```python
from build123d import *

# Parameters (mm, degrees)
BOSS_EXTRUDE1_DEPTH = 3
SKETCH3_W           = 12.065
SKETCH3_H           = 24.13
CUT_EXTRUDE1_DEPTH  = 114.708347838
CUT_EXTRUDE3_DEPTH  = 114.708347838
SKETCH5_R           = 0.8509
CUT_EXTRUDE4_DEPTH  = 114.708347838


with BuildPart() as part:
    # Sketch1 → Boss-Extrude1 (new body)
    with BuildSketch(Plane(origin=(0, 0, 0), x_dir=(1, 0, 0), z_dir=(0, 1, 0))):
        Polygon((0, 0), (0, 20.193), (-3, 20.193), (-3, 32.639), (0, 32.639), (0, 52.832), (41.783, 52.832), (41.783, 55.832), (54.229, 55.832), (54.229, 52.832), (96.012, 52.832), (96.012, 32.639), (99.012, 32.639), (99.012, 20.193), (96.012, 20.193), (96.012, 0), (54.229, 0), (54.229, -3), (41.783, -3), (41.783, 0), align=None)
    extrude(amount=BOSS_EXTRUDE1_DEPTH)

    # Sketch3 → Cut-Extrude1 (cut, through all)
    with BuildSketch(Plane(origin=(0, 3, 0), x_dir=(1, 0, 0), z_dir=(0, 1, 0))):
        with Locations((83.6295, 26.162)):
            Rectangle(SKETCH3_W, SKETCH3_H)
    extrude(amount=-CUT_EXTRUDE1_DEPTH, mode=Mode.SUBTRACT)

    # Sketch4 → Cut-Extrude3 (cut, through all)
    with BuildSketch(Plane(origin=(0, 3, 0), x_dir=(1, 0, 0), z_dir=(0, 1, 0))):
        with BuildLine():
            Line((96.012, 11.43), (96.012, 0))
            Line((96.012, 0), (84.582, 0))
            ThreePointArc((84.582, 0), (87.929769491, 8.082230509), (96.012, 11.43))
        make_face()
    extrude(amount=-CUT_EXTRUDE3_DEPTH, mode=Mode.SUBTRACT)

    # Sketch5 → Cut-Extrude4 (cut, through all)
    with BuildSketch(Plane(origin=(0, 3, 0), x_dir=(1, 0, 0), z_dir=(0, 1, 0))):
        with Locations(Location((83.8708, 39.9034, 0), (0, 0, 270))):
            Circle(SKETCH5_R)
        with Locations(Location((83.8708, 12.4206, 0), (0, 0, 270))):
            Circle(SKETCH5_R)
    extrude(amount=-CUT_EXTRUDE4_DEPTH, mode=Mode.SUBTRACT)


solid = part.part
```
Here's how the part is built. I have some questions about the finished solid (model axes, mm). A direction names the side the tool comes from. Coordinates: 2 decimals unless noted, no trailing zeros. Order: outer loops, then holes, each group sorted by start corner. A loop starts at its lowest first (then second) coordinate and runs counter-clockwise, first axis right, second up. Notation, with made-up numbers: M 62,50.25 L 112,50.25 A11 ccw 112,61.25 Z; hole C 32,19.5 d3. An arc over 180 degrees is marked long. Answer as a JSON object with one key per item and string values. Group by question number.
(1) Suppose I cut it at A-A, the plane z = -23.5. Please give me the cut outline in (x, y), then the cut area to 3 significant figures.
(2) Suppose I cut it at C-C, the plane x = 23.5. Please give me the cut outline in (y, z).
(3) Which directions (+Z, -Z, +X, -X, +Y, -Y) give clear straight access to the entire face, cutting with the end or side of a thin tool? Please do faces 1 (the face through (0, 1, -10)), 2 (the face through (98, 1, -20.193)), 3 (the face through (54.229, 1, -54)).
(4) For pin 1 (1.5 mm diameter, centred on y = 1, z = -12, fed in from -X); pin 2 (1 mm diameter, centred on x = 83.87, z = -39.9, fed in from -Y); pin 3 (0.9 mm diameter, centred on x = 72.5, y = 1.5, fed in from +Z); pin 4 (1.5 mm diameter, centred on y = 1, z = -46.5, fed in from +X), each with a flat end and sliding along its axis, tell me the tip position at first contact or that it passes through.
(5) Suppose I cut it at D-D, the plane z = -49. Please give me the cut outline in (x, y), then the cut area to 3 significant figures.
(6) I need wall thicknesses on probe 1 along X at (y, z) = (2.4, -34.5); probe 2 along X at (y, z) = (0.35, -27.5); probe 3 along Z at (x, y) = (78.5, 2.7). Which ranges of each line are inside material? Lowest first, please.
(7) Suppose I cut it at B-B, the plane y = 1.9. Please give me the cut outline in (x, z).
(8) If we mould it in two halves opening along Z, with no side actions, what happens to faces 4 (the face through (96.012, 1, -16)), 5 (the face through (84, 2, -38.227)), 6 (the face through (97, 1, -32.639))? For each: released by +Z, released by -Z, zero draft, split by the parting line, or undercut.
Values found:
{
 "1": {"outline": "M -3,0 L 77.6,0 L 77.6,3 L -3,3 Z; M 89.66,0 L 99.01,0 L 99.01,3 L 89.66,3 Z", "area": "270 mm^2"},
 "2": {"outline": "M 0,-52.83 L 3,-52.83 L 3,0 L 0,0 Z"},
 "3": {"face 1": "+Z, -X, +Y, -Y", "face 2": "+Z, +X, +Y, -Y", "face 3": "-Z, +X, +Y, -Y"},
 "4": {"pin 1": "stops at x = 0", "pin 2": "passes through", "pin 3": "stops at z = 0", "pin 4": "stops at x = 96.01"},
 "5": {"outline": "M 0,0 L 96.01,0 L 96.01,3 L 0,3 Z", "area": "288 mm^2"},
 "6": {"probe 1": "x = 0 to 77.6, 89.66 to 96.01", "probe 2": "x = -3 to 77.6, 89.66 to 99.01", "probe 3": "z = -52.83 to -38.23, -14.1 to 0"},
 "7": {"outline": "M -3,-32.64 L 0,-32.64 L 0,-52.83 L 41.78,-52.83 L 41.78,-55.83 L 54.23,-55.83 L 54.23,-52.83 L 96.01,-52.83 L 96.01,-32.64 L 99.01,-32.64 L 99.01,-20.19 L 96.01,-20.19 L 96.01,-11.43 A11.43 cw 84.58,0 L 54.23,0 L 54.23,3 L 41.78,3 L 41.78,0 L 0,0 L 0,-20.19 L -3,-20.19 Z; hole M 77.6,-38.23 L 89.66,-38.23 L 89.66,-14.1 L 77.6,-14.1 Z; hole C 83.87,-39.9 d1.7; hole C 83.87,-12.42 d1.7"},
 "8": {"face 4": "zero draft", "face 5": "undercut", "face 6": "released by -Z"}
}
